```python
from build123d import *

# Parameters (mm, degrees)
F1_DEPTH      = 4
F2_R          = 1
F3_DEPTH      = 5.001
F3_DEPTH_BACK = 5.001
F4_W          = 126
F4_H          = 10
F5_DEPTH      = 10
F6_SIZE2      = 2.99999
F6_SIZE       = 4.99999
F7_R          = 2
F8_R          = 1


# Not quite as in the source:
# - a fillet or chamfer is up to 0.001 mm smaller than in the source, because OpenCascade refuses the exact size


with BuildPart() as f1:
    # F0 (on Front) → F1 (new body, symmetric)
    with BuildSketch(Plane.XZ):
        Polygon((69, 2.25), (69, 5), (-69, 5), (-69, 2.25), (-61, 2.25), (-61, -2.25), (-69, -2.25), (-69, -5), (69, -5), (69, -2.25), (61, -2.25), (61, 2.25), align=None)
    extrude(amount=F1_DEPTH, both=True)

    # F2 (on Top) → F3 (cut, two sides)
    with BuildSketch(Plane.XY) as f3_sk:
        with Locations((-66.5, 0)):
            Circle(F2_R)
        with Locations((66.5, 0)):
            Circle(F2_R)
    extrude(amount=-F3_DEPTH, mode=Mode.SUBTRACT)
    extrude(f3_sk.sketch, amount=F3_DEPTH_BACK, mode=Mode.SUBTRACT)

    # F4 (on Top) → F5 (cut, symmetric)
    with BuildSketch(Plane.XY):
        with Locations((0, -6)):
            Rectangle(F4_W, F4_H)
    extrude(amount=F5_DEPTH, both=True, mode=Mode.SUBTRACT)

    # F6 (size 5 and 3 in the source; OpenCascade refuses exactly that, so slightly less here)
    f6_edges = [f1.edges().sort_by_distance(p)[0] for p in [
        (-63, -1, 3.625),
        (63, -1, 3.625),
    ]]
    f6_side = f1.faces().sort_by_distance((0, -1, 0))[0]
    chamfer(f6_edges, length=F6_SIZE, length2=F6_SIZE2, reference=f6_side)

    # F7
    f7_edges = [f1.edges().sort_by_distance(p)[0] for p in [
        (-69, 4, 3.625),
        (-69, 4, -3.625),
        (-69, -4, 3.625),
        (-69, -4, -3.625),
        (69, -4, 3.625),
        (69, -4, -3.625),
        (69, 4, -3.625),
        (69, 4, 3.625),
    ]]
    fillet(f7_edges, radius=F7_R)

    # F8
    f8_edges = [f1.edges().sort_by_distance(p)[0] for p in [
        (61, 0.600004, -2.25),
        (61, 0.600004, 2.25),
        (-61, 0.600004, 2.25),
        (-61, 0.600004, -2.25),
    ]]
    fillet(f8_edges, radius=F8_R)


solid = f1.part
```
Model file for the job. Use its own axes, mm. A direction names the side the tool comes from. Coordinates: 2 decimals unless noted, no trailing zeros. Order: outer loops, then holes, each group sorted by start corner. A loop starts at its lowest first (then second) coordinate and runs counter-clockwise, first axis right, second up. Notation, with made-up numbers: (-18, 14) -> (-1, 14) arc R21 cw to (-1, 48) -> close; hole circle Ø5 at (63.25, 67.25). An arc over 180 degrees is marked (long way). Answer as a JSON object with one key per item and string values. Group by question number.
1) Cut at A-A, the plane z = -3.75. Count the separate pieces of the cut face and the enclosed holes in it, then the cut area to 3 significant figures.
2) Drill centre lines: L1, parallel to X at y = 0, z = 2.5; L2, parallel to X at y = 0.5, z = 2.75; L3, parallel to Y at x = -66.5, z = -4.05. Where is each one in solid material? Low to high.
3) Which spindle directions (+Z, -Z, +X, -X, +Y, -Y) get a long thin tool onto all of the face, cutting with end or side? Do faces 4 (the face through (60, -2.2, 0.1)), 5 (the face through (-65, 0, -2.25)), 6 (the face through (65, 0, -2.25)). Say none if no direction does.
4) Cut at B-B, the plane x = -16. Write the cut outline in (y, z), then the cut area to 3 significant figures.
5) Flat gauge pins, fed straight in: pin 1 (2.5 mm diameter, centred on x = 66.5, y = 0, fed in from -Z); pin 2 (2 mm diameter, centred on y = 2, z = 0.5, fed in from -X); pin 3 (5 mm diameter, centred on x = -12.5, z = -0.5, fed in from -Y). Where does each tip first touch, or does it go through?
6) Pull direction Z, two halves, no side cores. Call faces 1 (the face through (65, 0, 2.25)), 2 (the face through (-1, 4, 0)), 3 (the face through (1, 1, 5)): +Z half, -Z half, draft (parallel to the pull), parting line (faces both ways), or undercut.
Check values:
{
 "1": {"separate pieces": "1", "enclosed holes": "2", "area": "731 mm²"},
 "2": {"L1": "x = -69 to -67.5, -65.5 to 65.5, 67.5 to 69", "L2": "x = -69 to -67.37, -65.63 to 65.63, 67.37 to 69", "L3": "y = -4 to -1, 1 to 4"},
 "3": {"face 4": "+Z, -Z, -Y", "face 5": "-X, +Y, -Y", "face 6": "+X, +Y, -Y"},
 "4": {"outline": "(-1, -5) -> (4, -5) -> (4, 5) -> (-1, 5) -> close", "area": "50.0 mm²"},
 "5": {"pin 1": "stops at z = -5", "pin 2": "stops at x = -61.03", "pin 3": "stops at y = -1"},
 "6": {"face 1": "undercut", "face 2": "draft", "face 3": "+Z half"}
}
